Part model, mm, in its own coordinate system. A direction names the side the tool comes from. Coordinates: 2 decimals unless noted, no trailing zeros. Loops run counter-clockwise (first coordinate to the right, second up) from the corner with the lowest first, then second, coordinate; pieces in that order, holes last. Notation, with made-up numbers: (-39, -11.5) -> (-27, -11.5) arc R21 cw to (-27, 9.5) -> close; hole circle Ø9 at (39.5, 57.25). An arc over 180 degrees is marked (long way). One line per question, with ' | ' between items. Start each with the question number.
1) 3-axis set-ups, long thin cutter, end or side, ignore diameter. For faces 4 (the face through (-8, 56, 8.667)), 5 (the face through (10, 54, -6)): which of +Z, -Z, +X, -X, +Y, -Y reach the whole face in a straight line?
2) Cut at B-B (z = 0). List the corners of the cut face in (x, y).
3) Cut at A-A (x = 0). List the corners of the cut face in (y, z), plus the area to 3 significant figures.
4) Cut at C-C (y = 71.5). Count the separate pieces of the cut face and the enclosed holes in it, plus the area to 3 significant figures.
5) Drop flat-ended pins along their axis: pin 1 (12 mm diameter, centred on x = 4, z = -7.5, fed in from +Y); pin 2 (1.1 mm diameter, centred on x = -9.5, y = 35, fed in from -Z). Give the stop position or say it passes through.
6) Two-plate mould, pull along Z, no slides. Class faces 1 (the face through (2, 0, 2)), 2 (the face through (8, 56, 6.8)), 3 (the face through (-6, 54, 10)): released by +Z, released by -Z, zero draft, split by the parting line, or undercut.
7) Probe L1, parallel to Z at x = -7.25, y = 60; L2, parallel to Y at x = 0.75, z = 3.25. List the from-to ranges inside material, lowest first. Write a range as from..to.
from build123d import *

# Parameters (mm, degrees)
SKETCH1_W           = 20
SKETCH1_H           = 20
EXTRUDE1_DEPTH      = 110
SKETCH2_R           = 2.266666667
SKETCH2_W           = 1.866666667
SKETCH2_H           = 1.866666667
EXTRUDE2_DEPTH      = 111.905365064
FILLET1_R           = 1.333333333
SKETCH_3_W          = 5
SKETCH_3_H          = 5
CUT_EXTRUDE_1_DEPTH = 10


with BuildPart() as part:
    # Sketch1 → Extrude1 (new body)
    with BuildSketch(Plane(origin=(0, 0, 0), x_dir=(1, 0, 0), z_dir=(0, 1, 0))):
        Rectangle(SKETCH1_W, SKETCH1_H)
    extrude(amount=EXTRUDE1_DEPTH)

    # Sketch2 → Extrude2 (cut, through all)
    with BuildSketch(Plane(origin=(0, 110, 0), x_dir=(1, 0, 0), z_dir=(0, 1, 0))):
        with Locations(Location((0, 0, 0), (0, 0, 270))):
            Circle(SKETCH2_R)
        Polygon((8.666666667, 3), (11.333333333, 3), (11.333333333, -3), (8.666666667, -3), (8.666666667, -5.466666667), (6.409475708, -5.466666667), (4.133333333, -3.190524292), (4.133333333, 3.190524292), (6.409475708, 5.466666667), (8.666666667, 5.466666667), align=None)
        with Locations((7.733333334, 7.733333334)):
            Rectangle(SKETCH2_W, SKETCH2_H)
        Polygon((-3.190524292, 4.133333333), (-5.466666667, 6.409475708), (-5.466666667, 8.666666667), (-3, 8.666666667), (-3, 11.333333333), (3, 11.333333333), (3, 8.666666667), (5.466666667, 8.666666667), (5.466666667, 6.409475708), (3.190524292, 4.133333333), align=None)
        with Locations((7.733333334, -7.733333334)):
            Rectangle(SKETCH2_W, SKETCH2_H)
        with Locations((-7.733333334, 7.733333334)):
            Rectangle(SKETCH2_W, SKETCH2_H)
        with Locations((-7.733333334, -7.733333334)):
            Rectangle(SKETCH2_W, SKETCH2_H)
        Polygon((-6.409475708, -5.466666667), (-8.666666667, -5.466666667), (-8.666666667, -3), (-11.333333333, -3), (-11.333333333, 3), (-8.666666667, 3), (-8.666666667, 5.466666667), (-6.409475708, 5.466666667), (-4.133333333, 3.190524292), (-4.133333333, -3.190524292), align=None)
        Polygon((3.190524292, -4.133333333), (-3.190524292, -4.133333333), (-5.466666667, -6.409475708), (-5.466666667, -8.666666667), (-3, -8.666666667), (-3, -11.333333333), (3, -11.333333333), (3, -8.666666667), (5.466666667, -8.666666667), (5.466666667, -6.409475708), align=None)
    extrude(amount=-EXTRUDE2_DEPTH, mode=Mode.SUBTRACT)

    # Fillet1
    fillet1_edges = [part.edges().sort_by_distance(p)[0] for p in [
        (10, 55, 10),
        (-10, 55, 10),
        (-10, 55, -10),
        (10, 55, -10),
    ]]
    fillet(fillet1_edges, radius=FILLET1_R)

    # Sketch 3 → Cut-Extrude 1 (cut, symmetric)
    with BuildSketch(Plane.XY):
        with Locations((0, 55)):
            Rectangle(SKETCH_3_W, SKETCH_3_H)
    extrude(amount=CUT_EXTRUDE_1_DEPTH, both=True, mode=Mode.SUBTRACT)


solid = part.part
Reported:
1) face 4: +Y, -Y | face 5: +Z, -Z, +X, +Y, -Y
2) outline: (-4.13, 0) -> (-2.27, 0) -> (-2.27, 52.5) -> (-2.5, 52.5) -> (-2.5, 57.5) -> (-2.27, 57.5) -> (-2.27, 110) -> (-4.13, 110) -> close; (2.27, 0) -> (4.13, 0) -> (4.13, 110) -> (2.27, 110) -> (2.27, 57.5) -> (2.5, 57.5) -> (2.5, 52.5) -> (2.27, 52.5) -> close
3) outline: (0, -4.13) -> (52.5, -4.13) -> (52.5, -2.27) -> (0, -2.27) -> close; (0, 2.27) -> (52.5, 2.27) -> (52.5, 4.13) -> (0, 4.13) -> close; (57.5, -4.13) -> (110, -4.13) -> (110, -2.27) -> (57.5, -2.27) -> close; (57.5, 2.27) -> (110, 2.27) -> (110, 4.13) -> (57.5, 4.13) -> close | area: 392 mm²
4) separate pieces: 1 | enclosed holes: 5 | area: 159 mm²
5) pin 1: stops at y = 110 | pin 2: stops at z = -9.97
6) face 1: zero draft | face 2: undercut | face 3: released by +Z
7) L1: z = -10..-8.67, -6.8..-5.47, 5.47..6.8, 8.67..10 | L2: y = 0..52.5, 57.5..110
